Work out the finished part from the listing and answer in its coordinate system (mm). Round coordinates to 2 decimals unless told otherwise and drop trailing zeros. Loops run counter-clockwise (first coordinate to the right, second up) from the corner with the lowest first, then second, coordinate; pieces in that order, holes last.
```python
from build123d import *

# Parameters (mm, degrees)
SKETCH1_R           = 1.5
SKETCH1_W           = 196.314766664
SKETCH1_H           = 196.314766664
BOSS_EXTRUDE1_DEPTH = 4
SKETCH7_W           = 110.317049386
SKETCH7_H           = 4
CUT_EXTRUDE1_DEPTH  = 10
FILLET1_R           = 4


with BuildPart() as part:
    # Sketch1 → Boss-Extrude1 (new body)
    with BuildSketch(Plane(origin=(0, 0, 0), x_dir=(1, 0, 0), z_dir=(0, 1, 0))):
        Polygon((154.855, -139.95), (165.325, -139.95), (165.325, 139.95), (154.855, 139.95), (154.855, 143.95), (138.875, 143.95), (138.875, 128.61722325), (132.375, 124.864446501), (125.875, 128.61722325), (125.875, 143.95), (-125.875, 143.95), (-125.875, 128.61722325), (-132.375, 124.864446501), (-138.875, 128.61722325), (-138.875, 143.95), (-154.855, 143.95), (-154.855, 139.95), (-165.325, 139.95), (-165.325, -139.95), (-154.855, -139.95), (-154.855, -143.95), (-138.875, -143.95), (-138.875, -128.61722325), (-132.375, -124.864446501), (-125.875, -128.61722325), (-125.875, -143.95), (125.875, -143.95), (125.875, -128.61722325), (132.375, -124.864446501), (138.875, -128.61722325), (138.875, -143.95), (154.855, -143.95), align=None)
        with Locations(Location((-147.795, -135.95, 0), (0, 0, 270))):
            Circle(SKETCH1_R, mode=Mode.SUBTRACT)
        with Locations(Location((-119.795, -135.95, 0), (0, 0, 270))):
            Circle(SKETCH1_R, mode=Mode.SUBTRACT)
        with Locations(Location((-104.5, -104.5, 0), (0, 0, 270))):
            Circle(SKETCH1_R, mode=Mode.SUBTRACT)
        with Locations(Location((119.795, -135.95, 0), (0, 0, 270))):
            Circle(SKETCH1_R, mode=Mode.SUBTRACT)
        with Locations(Location((147.795, -135.95, 0), (0, 0, 270))):
            Circle(SKETCH1_R, mode=Mode.SUBTRACT)
        with Locations(Location((104.5, -104.5, 0), (0, 0, 270))):
            Circle(SKETCH1_R, mode=Mode.SUBTRACT)
        with Locations(Location((-104.5, 104.5, 0), (0, 0, 270))):
            Circle(SKETCH1_R, mode=Mode.SUBTRACT)
        with Locations(Location((-147.795, 135.95, 0), (0, 0, 270))):
            Circle(SKETCH1_R, mode=Mode.SUBTRACT)
        with Locations(Location((-119.795, 135.95, 0), (0, 0, 270))):
            Circle(SKETCH1_R, mode=Mode.SUBTRACT)
        Rectangle(SKETCH1_W, SKETCH1_H, mode=Mode.SUBTRACT)
        with Locations(Location((104.5, 104.5, 0), (0, 0, 270))):
            Circle(SKETCH1_R, mode=Mode.SUBTRACT)
        with Locations(Location((86.915968312, 117.1513625, 0), (0, 0, 270))):
            Circle(SKETCH1_R, mode=Mode.SUBTRACT)
        with Locations(Location((101.875, 117.1513625, 0), (0, 0, 270))):
            Circle(SKETCH1_R, mode=Mode.SUBTRACT)
        with Locations(Location((86.915968312, 133.95, 0), (0, 0, 270))):
            Circle(SKETCH1_R, mode=Mode.SUBTRACT)
        with Locations(Location((101.875, 133.95, 0), (0, 0, 270))):
            Circle(SKETCH1_R, mode=Mode.SUBTRACT)
        with Locations(Location((119.795, 135.95, 0), (0, 0, 270))):
            Circle(SKETCH1_R, mode=Mode.SUBTRACT)
        with Locations(Location((147.795, 135.95, 0), (0, 0, 270))):
            Circle(SKETCH1_R, mode=Mode.SUBTRACT)
    extrude(amount=BOSS_EXTRUDE1_DEPTH)

    # Sketch7 → Cut-Extrude1 (cut)
    with BuildSketch(Plane.ZY.offset(-98.157383332)):
        with Locations((-1.45907227, 2)):
            Rectangle(SKETCH7_W, SKETCH7_H)
    extrude(amount=-CUT_EXTRUDE1_DEPTH, mode=Mode.SUBTRACT)

    # Fillet1
    fillet1_edges = [part.edges().sort_by_distance(p)[0] for p in [
        (108.157383332, 2, -56.617596963),
        (108.157383332, 2, 53.699452423),
        (98.157383332, 2, -56.617596963),
        (98.157383332, 2, 53.699452423),
    ]]
    fillet(fillet1_edges, radius=FILLET1_R)


solid = part.part
```
1. Given pin 1 (2.5 mm diameter, centred on x = -119.795, z = -135.95, fed in from +Y); pin 2 (1.2 mm diameter, centred on x = 162.5, y = 2, fed in from -Z); pin 3 (2 mm diameter, centred on y = 2, z = -141, fed in from +X) (3 decimals); pin 4 (2 mm diameter, centred on x = 162.5, y = 1, fed in from +Z), each flat-ended and moving along its own axis, determine where each tip first touches the part or whether it passes through.
Answer key:
pin 1: passes through
pin 2: stops at z = -139.95
pin 3: stops at x = 154.855
pin 4: stops at z = 139.95
2. Find section C-C (y = 3.3). Give the number of separate pieces and of enclosed holes in the cut face, then the cut area to 3 significant figures.
Answer key:
separate pieces: 1
enclosed holes: 17
area: 54,400 mm2
3. Find section A-A (z = -42.5). Write down the section's boundary in (x, y) (3 decimals).
Answer key:
outline: (-165.325, 0) - (-98.157, 0) - (-98.157, 4) - (-165.325, 4) - close; (108.157, 0) - (165.325, 0) - (165.325, 4) - (108.157, 4) - close
4. Consider probe 1 along Z at (x, y) = (104.5, 0.95); probe 2 along Z at (x, y) = (104, 1.2); probe 3 along X at (y, z) = (1.35, -133.95) (3 decimals). Determine where each line is inside the solid, lowest interval first.
Answer key:
probe 1: z = -143.95 to -106, -103 to -56.6, 53.68 to 103, 106 to 143.95
probe 2: z = -143.95 to -105.91, -103.09 to -56.62, 53.7 to 103.09, 105.91 to 143.95
probe 3: x = -165.325 to -138.875, -125.875 to 85.416, 88.416 to 100.375, 103.375 to 125.875, 138.875 to 165.325
5. Find section B-B (x = -41). Write down the section's boundary in (y, z).
Answer key:
outline: (0, -143.95) - (4, -143.95) - (4, -98.16) - (0, -98.16) - close; (0, 98.16) - (4, 98.16) - (4, 143.95) - (0, 143.95) - close
